from build123d import *

# Parameters (mm, degrees)
SKETCH1_W               = 311.094159216
SKETCH1_H               = 144.015986956
BOSS_EXTRUDE1_DEPTH     = 10
SKETCH2_R               = 11.561372413
CUT_EXTRUDE1_DEPTH      = 10
FILL_PATTERN1_OUTLINE_R = 11.561372413
FILL_PATTERN1_DEPTH     = 10


# Read off the part's stored shape, not the designer's step: Fill Pattern1
with BuildPart() as part:
    # Sketch1 → Boss-Extrude1 (new body)
    with BuildSketch(Plane(origin=(0, 0, 0), x_dir=(1, 0, 0), z_dir=(0, 1, 0))):
        Rectangle(SKETCH1_W, SKETCH1_H)
    extrude(amount=BOSS_EXTRUDE1_DEPTH)

    # Sketch2 → Cut-Extrude1 (cut)
    with BuildSketch(Plane(origin=(0, 10, 0), x_dir=(1, 0, 0), z_dir=(0, 1, 0))):
        with Locations(Location((0, 0, 0), (0, 0, 270))):
            Circle(SKETCH2_R)
    extrude(amount=-CUT_EXTRUDE1_DEPTH, mode=Mode.SUBTRACT)

    # Fill Pattern1 outline → Fill Pattern1 (cut)
    with BuildSketch(Plane(origin=(0, 0, 0), x_dir=(1, 0, 0), z_dir=(0, 1, 0))):
        with Locations((-120.173715992, -1.428513712)):
            Circle(FILL_PATTERN1_OUTLINE_R)
        with Locations((80.683289444, -46.786810115)):
            Circle(FILL_PATTERN1_OUTLINE_R)
        with Locations((99.861023935, 25.060004388)):
            Circle(FILL_PATTERN1_OUTLINE_R)
        with Locations((80.115810661, 0.952342474)):
            Circle(FILL_PATTERN1_OUTLINE_R)
        with Locations((60.370597387, -23.155319439)):
            Circle(FILL_PATTERN1_OUTLINE_R)
        with Locations((100.428502718, -22.679148202)):
            Circle(FILL_PATTERN1_OUTLINE_R)
        with Locations((120.173715992, 1.428513712)):
            Circle(FILL_PATTERN1_OUTLINE_R)
        with Locations((-20.312692057, 23.631490676)):
            Circle(FILL_PATTERN1_OUTLINE_R)
        with Locations((-40.057905331, -0.476171237)):
            Circle(FILL_PATTERN1_OUTLINE_R)
        with Locations((-59.803118605, -24.583833151)):
            Circle(FILL_PATTERN1_OUTLINE_R)
        with Locations((-79.548331879, -48.691495064)):
            Circle(FILL_PATTERN1_OUTLINE_R)
        with Locations((-100.428502718, 22.679148202)):
            Circle(FILL_PATTERN1_OUTLINE_R)
        with Locations((-99.861023935, -25.060004388)):
            Circle(FILL_PATTERN1_OUTLINE_R)
        with Locations((-80.115810661, -0.952342474)):
            Circle(FILL_PATTERN1_OUTLINE_R)
        with Locations((-60.370597387, 23.155319439)):
            Circle(FILL_PATTERN1_OUTLINE_R)
        with Locations((20.312692057, -23.631490676)):
            Circle(FILL_PATTERN1_OUTLINE_R)
        with Locations((40.057905331, 0.476171237)):
            Circle(FILL_PATTERN1_OUTLINE_R)
        with Locations((59.803118605, 24.583833151)):
            Circle(FILL_PATTERN1_OUTLINE_R)
        with Locations((40.625384113, -47.262981352)):
            Circle(FILL_PATTERN1_OUTLINE_R)
        with Locations((-39.490426548, -48.215323827)):
            Circle(FILL_PATTERN1_OUTLINE_R)
        with Locations((-19.745213274, -24.107661913)):
            Circle(FILL_PATTERN1_OUTLINE_R)
        with Locations((19.745213274, 24.107661913)):
            Circle(FILL_PATTERN1_OUTLINE_R)
        with Locations((0.567478783, -47.73915259)):
            Circle(FILL_PATTERN1_OUTLINE_R)
    extrude(amount=FILL_PATTERN1_DEPTH, mode=Mode.SUBTRACT)


solid = part.part
Input: part model. Units: mm. Frame: model coordinates. Round coordinates to 2 decimals unless told otherwise and drop trailing zeros. Order: outer loops, then holes, each group sorted by start corner. A loop starts at its lowest first (then second) coordinate and runs counter-clockwise, first axis right, second up.
1. Pin query (flat end, axial travel): P1, Ø14, axis at x = -80.12, z = 0.95, coming from the +Y side; P2, Ø8, axis at x = -47.5, z = 19, coming from the -Y side. Return the tip coordinate at first contact, or that it passes through.
The answers:
P1: passes through
P2: stops at y = 0
2. Cut plane B-B, the plane y = 4.75. State how many separate pieces and enclosed holes the cut face has, then the cut area to 3 significant figures.
The answers:
separate pieces: 1
enclosed holes: 24
area: 34,700 mm2
3. Cut plane C-C, the plane x = 97.5. Output: boundary loops of the cut face in (y, z), then the cut area to 3 significant figures.
The answers:
outline: (0, -72.01) - (10, -72.01) - (10, -36.38) - (0, -36.38) - close; (0, -13.74) - (10, -13.74) - (10, 11.49) - (0, 11.49) - close; (0, 33.86) - (10, 33.86) - (10, 72.01) - (0, 72.01) - close
area: 990 mm2
4. Material intervals for line 1 (Z direction, x = 20, y = 0.75); line 2 (X direction, y = 9, z = 42); line 3 (Z direction, x = 68.5, y = 4), sorted ascending.
The answers:
line 1: z = -72.01 to -35.67, -12.55 to 12.07, 35.19 to 72.01
line 2: x = -155.55 to -88.98, -70.12 to -49.24, -29.74 to -9.47, 10.6 to 30.33, 50.92 to 70.16, 91.21 to 155.55
line 3: z = -72.01 to -32.2, -16.97 to 14.93, 31.38 to 72.01
5. Mould query, pull axis X, two halves, no side actions, for faces 1 (the face through (-22.251, 4.93, 35.394)), 2 (the face through (-2, 5, 72.008)), 3 (the face through (-155.547, 5, 1)), 4 (the face through (50.63, 4.93, -17.55)). Classes: released by +X, released by -X, zero draft, split by the parting line, or undercut.
The answers:
face 1: undercut
face 2: zero draft
face 3: released by -X
face 4: undercut
6. Cut plane A-A, the plane x = 23. Output: boundary loops of the cut face in (y, z).
The answers:
outline: (0, -72.01) - (10, -72.01) - (10, -35.2) - (0, -35.2) - close; (0, -13.01) - (10, -13.01) - (10, 12.39) - (0, 12.39) - close; (0, 34.88) - (10, 34.88) - (10, 72.01) - (0, 72.01) - close
